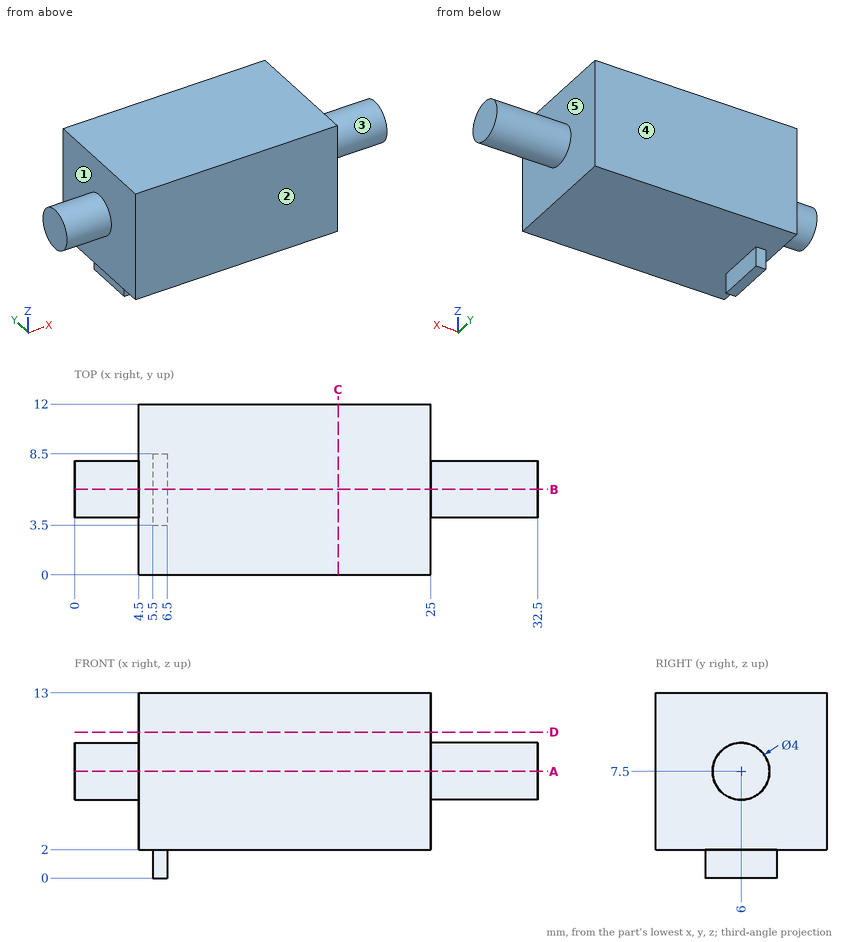
Input: dimensioned drawing with shaded views. Units: mm. Origin: part minimum x, y, z. A direction names the side the tool comes from. Give positions to 0.01 mm unless a question says otherwise; leave off trailing zeros. Loops run counter-clockwise (first coordinate to the right, second up) from the corner with the lowest first, then second, coordinate; pieces in that order, holes last. Notation, with made-up numbers: M -7,26 L 44,26 A21 cw 44,32 Z; hole C 87,-39.5 d7. An arc over 180 degrees is marked long. Put each result on its own line as item: value. Start each with the question number.
1) Cut plane B-B (y = 6). Output: boundary loops of the cut face in (x, z).
2) Cut plane C-C (x = 18.5). Output: boundary loops of the cut face in (y, z), then the cut area to 3 significant figures.
3) Contact query for flat-ended pins moving along their axis: pin 1 (0.8 mm diameter, centred on x = 6, z = 1.5, fed in from +Y); pin 2 (2 mm diameter, centred on x = 22, z = 5.5, fed in from -Y); pin 3 (2 mm diameter, centred on y = 5.5, z = 2.5, fed in from -X); pin 4 (3.5 mm diameter, centred on x = 19, y = 8, fed in from -Z). Output: stop coordinate, or through.
4) Cut plane A-A (z = 7.5). Output: boundary loops of the cut face in (x, y), then the cut area to 3 significant figures.
5) Access query for the marked faces 1 and 2. Directions: +Z, -Z, +X, -X, +Y, -Y. A direction counts if a zero-diameter tool reaches every point of the face in a straight line with its end or side. Return the directions, or none.
6) Ray query, line 1 along X through (y, z) = (11.5, 8.5); line 2 along Z through (x, y) = (22, 5.75); line 3 along X through (y, z) = (5.75, 1.75). Return the intervals inside material, ascending.
7) Pull-direction query (Y, two-part tool) for the marked faces 3, 4 and 5; classes: pulls with the +Y half, pulls with the -Y half, needs draft (parallel to the pull), parting line crosses it, or undercut.
8) Cut plane D-D (z = 10.25). Output: boundary loops of the cut face in (x, y), then the cut area to 3 significant figures.
Verdict:
1. outline: M 0,5.5 L 4.5,5.5 L 4.5,2 L 5.5,2 L 5.5,0 L 6.5,0 L 6.5,2 L 25,2 L 25,5.5 L 32.5,5.5 L 32.5,9.5 L 25,9.5 L 25,13 L 4.5,13 L 4.5,9.5 L 0,9.5 Z
2. outline: M 0,2 L 12,2 L 12,13 L 0,13 Z
2. area: 132 mm2
3. pin 1: y = 8.5
3. pin 2: y = 0
3. pin 3: x = 4.5
3. pin 4: z = 2
4. outline: M 0,4 L 4.5,4 L 4.5,0 L 25,0 L 25,4 L 32.5,4 L 32.5,8 L 25,8 L 25,12 L 4.5,12 L 4.5,8 L 0,8 Z
4. area: 294 mm2
5. face 1: -X
5. face 2: +Z, -Z, +X, -X, -Y
6. line 1: 4.5 to 25
6. line 2: 2 to 13
6. line 3: 5.5 to 6.5
7. face 3: parting line crosses it
7. face 4: pulls with the +Y half
7. face 5: needs draft
8. outline: M 4.5,0 L 25,0 L 25,12 L 4.5,12 Z
8. area: 246 mm2
